from build123d import *

# Parameters (mm, degrees)
F1_DEPTH = 12.7
F0_W     = 93.1164
F0_H     = 152.805166
F2_DEPTH = 23.2918
F3_R     = 5.08
F4_W     = 76.2
F4_H     = 0.0508
F5_DEPTH = 2.159
F6_W     = 76.2
F6_H     = 0.0508
F7_DEPTH = 2.159


with BuildPart() as f1:
    # F0 (on Top) → F1 (new body)
    with BuildSketch(Plane.XY):
        with BuildLine():
            Line((33.8582, -61.6204), (33.8582, 61.6204))
            ThreePointArc((33.8582, 61.6204), (0, 63.702583), (-33.8582, 61.6204))
            Line((-33.8582, 61.6204), (-33.8582, -61.6204))
            ThreePointArc((-33.8582, -61.6204), (0, -63.702583), (33.8582, -61.6204))
        make_face()
    extrude(amount=F1_DEPTH)

    # F0 (on Top) → F2 (join)
    with BuildSketch(Plane.XY):
        Rectangle(F0_W, F0_H)
        with BuildLine():
            ThreePointArc((-33.8582, 61.6204), (0, 63.702583), (33.8582, 61.6204))
            Line((33.8582, 61.6204), (33.8582, -61.6204))
            ThreePointArc((33.8582, -61.6204), (0, -63.702583), (-33.8582, -61.6204))
            Line((-33.8582, -61.6204), (-33.8582, 61.6204))
        make_face(mode=Mode.SUBTRACT)
    extrude(amount=F2_DEPTH)

    # F3
    f3_edges = [f1.edges().sort_by_distance(p)[0] for p in [
        (46.5582, 76.402583, 11.6459),
        (-46.5582, 76.402583, 11.6459),
        (0, 76.402583, 0),
        (0, 76.402583, 23.2918),
        (46.5582, -76.402583, 11.6459),
        (46.5582, 0, 0),
        (46.5582, 0, 23.2918),
        (-46.5582, -76.402583, 11.6459),
        (-46.5582, 0, 0),
        (-46.5582, 0, 23.2918),
        (0, -76.402583, 0),
        (0, -76.402583, 23.2918),
    ]]
    fillet(f3_edges, radius=F3_R)

    # F4 (on face) → F5 (join)
    with BuildSketch(Plane.YZ.offset(-33.8582)):
        with Locations((0.031095, 23.2664)):
            Rectangle(F4_W, F4_H)
    extrude(amount=F5_DEPTH)

    # F6 (on face) → F7 (join)
    with BuildSketch(Plane(origin=(33.8582, 0, 0), x_dir=(0, -1, 0), z_dir=(-1, 0, 0))):
        with Locations((0, 23.2664)):
            Rectangle(F6_W, F6_H)
    extrude(amount=F7_DEPTH)


solid = f1.part
Input: part model. Units: mm. Frame: model coordinates. A direction names the side the tool comes from. Coordinates: 2 decimals unless noted, no trailing zeros. Loops run counter-clockwise (first coordinate to the right, second up) from the corner with the lowest first, then second, coordinate; pieces in that order, holes last.
Q1. Set-up query: faces 4 (the face through (0.475, -63.702, 17.922)), 5 (the face through (-1, 76.403, 12)). Return all of +Z, -Z, +X, -X, +Y, -Y with unobstructed straight access to the full face (end or side cutting, diameter ignored); none if empty.
Q2. Cut plane D-D (z = 21.75). Output: boundary loops of the cut face in (x, y).
Q3. Draft query along Y for faces 1 (the face through (-45.11, 74.875, 11.738)), 2 (the face through (-33.858, -1, 18)), 3 (the face through (45.031, 0.999, 21.843)). Return one class per face: +Y half, -Y half, draft (parallel to the pull), parting line (faces both ways), or undercut.
Q4. Contact query for flat-ended pins moving along their axis: pin 1 (4 mm diameter, centred on x = -28, y = -40, fed in from +Z); pin 2 (3 mm diameter, centred on y = 1, z = 20.5, fed in from -X); pin 3 (2 mm diameter, centred on x = 16.5, z = 21, fed in from +Y). Output: stop coordinate, or through.
Q5. Cut plane C-C (x = 3). Output: boundary loops of the cut face in (y, z), then the cut area to 3 significant figures.
Q6. Cut plane B-B (y = -5). Output: boundary loops of the cut face in (x, z), then the cut area to 3 significant figures.
Q7. Cut plane A-A (z = 15). Output: boundary loops of the cut face in (x, y), then the cut area to 3 significant figures.
Q8. Material intervals for line 1 (X direction, y = -54, z = 18.25); line 2 (Z direction, x = 7, y = 61.5); line 3 (X direction, y = 58.5, z = 20.5), sorted ascending.
Working result:
1. face 4: +Z
1. face 5: +Z, -Z, +X, -X, +Y
2. outline: (-45.12, -71.32) arc R3.65 ccw to (-41.48, -74.97) - (41.48, -74.97) arc R3.65 ccw to (45.12, -71.32) - (45.12, 71.32) arc R3.65 ccw to (41.48, 74.97) - (-41.48, 74.97) arc R3.65 ccw to (-45.12, 71.32) - close; hole (-33.86, -61.62) arc R276.32 ccw to (33.86, -61.62) - (33.86, 61.62) arc R276.32 ccw to (-33.86, 61.62) - close
3. face 1: +Y half
3. face 2: undercut
3. face 3: draft
4. pin 1: stops at z = 12.7
4. pin 2: stops at x = -46.5
4. pin 3: stops at y = 76.08
5. outline: (-76.4, 5.08) arc R5.08 ccw to (-71.32, 0) - (71.32, 0) arc R5.08 ccw to (76.4, 5.08) - (76.4, 18.21) arc R5.08 ccw to (71.32, 23.29) - (63.69, 23.29) - (63.69, 12.7) - (-63.69, 12.7) - (-63.69, 23.29) - (-71.32, 23.29) arc R5.08 ccw to (-76.4, 18.21) - close
5. area: 2,190 mm2
6. outline: (-46.56, 5.08) arc R5.08 ccw to (-41.48, 0) - (41.48, 0) arc R5.08 ccw to (46.56, 5.08) - (46.56, 18.21) arc R5.08 ccw to (41.48, 23.29) - (31.7, 23.29) - (31.7, 23.24) - (33.86, 23.24) - (33.86, 12.7) - (-33.86, 12.7) - (-33.86, 23.24) - (-31.7, 23.24) - (-31.7, 23.29) - (-41.48, 23.29) arc R5.08 ccw to (-46.56, 18.21) - close
6. area: 1,430 mm2
7. outline: (-46.56, -71.32) arc R5.08 ccw to (-41.48, -76.4) - (41.48, -76.4) arc R5.08 ccw to (46.56, -71.32) - (46.56, 71.32) arc R5.08 ccw to (41.48, 76.4) - (-41.48, 76.4) arc R5.08 ccw to (-46.56, 71.32) - close; hole (-33.86, -61.62) arc R276.32 ccw to (33.86, -61.62) - (33.86, 61.62) arc R276.32 ccw to (-33.86, 61.62) - close
7. area: 5,670 mm2
8. line 1: x = -46.56 to -33.86, 33.86 to 46.56
8. line 2: z = 0 to 12.7
8. line 3: x = -46.01 to -33.86, 33.86 to 46.01
